from build123d import *

# Parameters (mm, degrees)
PAD_DEPTH    = 2
SKETCH001_R  = 2
POCKET_DEPTH = 2.001


with BuildPart() as part:
    # Sketch → Pad (new body)
    with BuildSketch(Plane.XY):
        with BuildLine():
            Line((0, 4), (-9.650421, 4))
            ThreePointArc((-9.650421, -4), (-9.212813, 0), (-9.650421, 4))
            Line((-9.650421, -4), (0, -4))
            ThreePointArc((0, -4), (0.287187, 0), (0, 4))
        make_face()
    extrude(amount=PAD_DEPTH)

    # Sketch001 (on Face6 of Pad) → Pocket (cut, through all)
    with BuildSketch(Plane.XY.offset(2)):
        with Locations((-2.712813, 0)):
            Circle(SKETCH001_R)
    extrude(amount=-POCKET_DEPTH, mode=Mode.SUBTRACT)


solid = part.part
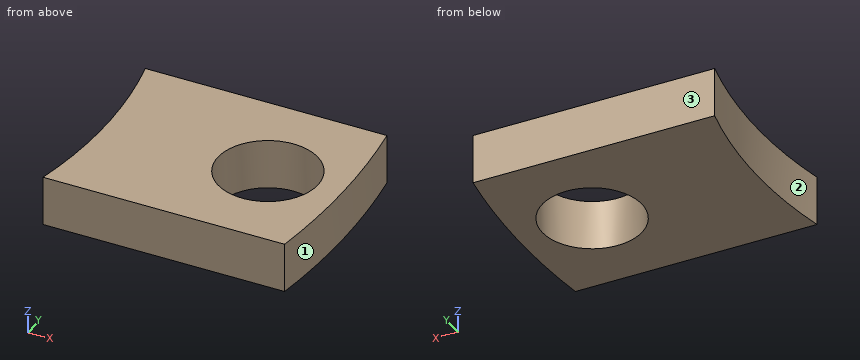
Model file for the job. Use its own axes, mm. Face numbers are marked on the shaded views. Round coordinates to 2 decimals unless told otherwise and drop trailing zeros. Loops run counter-clockwise (first coordinate to the right, second up) from the corner with the lowest first, then second, coordinate; pieces in that order, holes last.
1. Mould opens along Y. For the marked faces 1, 2 and 3 say: +Y half, -Y half, draft (parallel to the pull), parting line (faces both ways), or undercut.
Check values:
face 1: parting line
face 2: undercut
face 3: +Y half
2. Band-saw the part on D-D, the plane y = 3.25. List the corners of the cut face in (x, z), and give its area (3 significant figures).
Check values:
outline: (-9.5, 0) - (0.1, 0) - (0.1, 2) - (-9.5, 2) - close
area: 19.2 mm2
3. Drop a flat-ended pin along its axis: P1, Ø3, axis at x = -2.71, y = 0, coming from the +Z side. Give the stop position or say it passes through.
Check values:
P1: passes through
4. Wall check: probe 1 along Y at (x, z) = (-2.75, 1.2); probe 2 along X at (y, z) = (-0.25, 1.35); probe 3 along X at (y, z) = (-0.75, 0.8). Give the ranges that are in metal, low to high.
Check values:
probe 1: y = -4 to -2, 2 to 4
probe 2: x = -9.21 to -4.7, -0.73 to 0.29
probe 3: x = -9.23 to -4.57, -0.86 to 0.28
5. Band-saw the part on A-A, the plane y = 0. List the corners of the cut face in (x, z).
Check values:
outline: (-9.21, 0) - (-4.71, 0) - (-4.71, 2) - (-9.21, 2) - close; (-0.71, 0) - (0.29, 0) - (0.29, 2) - (-0.71, 2) - close
6. Band-saw the part on C-C, the plane z = 0.9. List the corners of the cut face in (x, y), and give its area (3 significant figures).
Check values:
outline: (-9.65, -4) - (0, -4) arc R28 ccw to (0, 4) - (-9.65, 4) arc R18.5 cw to start; hole circle Ø4 at (-2.71, 0)
area: 63.8 mm2
7. Band-saw the part on B-B, the plane x = -4.5. List the corners of the cut face in (y, z).
Check values:
outline: (-4, 0) - (-0.9, 0) - (-0.9, 2) - (-4, 2) - close; (0.9, 0) - (4, 0) - (4, 2) - (0.9, 2) - close
